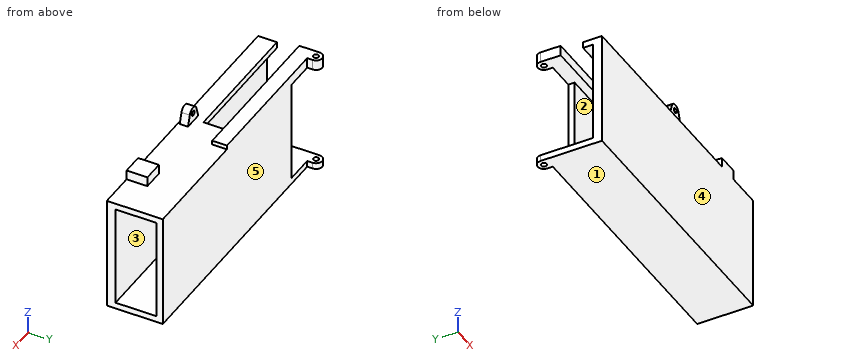
from build123d import *

# Parameters (mm, degrees)
SKETCH_1_W               = 27.5
SKETCH_1_H               = 10.9
SKETCH_1_W_2             = 24.5
SKETCH_1_H_2             = 7.9
EXTRUDE_1_DEPTH          = 66
SKETCH_3_W               = 141.586461115
SKETCH_3_H               = 11.077241851
CUT_EXTRUDE_1_DEPTH      = 50
SKETCH_4_R               = 0.65
EXTRUDE_2_DEPTH          = 27.5
CUT_EXTRUDE_2_DEPTH      = 10
CUT_EXTRUDE_2_DEPTH_BACK = 10
SKETCH_5_W               = 27.947827097
SKETCH_5_H               = 24.5
EXTRUDE_3_DEPTH          = 66
EXTRUDE_START            = -11
SKETCH_9_R               = 0.6
EXTRUDE_5_DEPTH          = 2
SKETCH_10_W              = 33.442715753
SKETCH_10_H              = 5.368535072
CUT_EXTRUDE_3_DEPTH      = 2.6
SKETCH_11_W              = 5
SKETCH_11_H              = 2.3
EXTRUDE_6_DEPTH          = 5
EXTRUDE_START_2          = 1
SKETCH_12_R              = 0.65
EXTRUDE_7_DEPTH          = 1
SKETCH_13_W              = 24.5
SKETCH_13_H              = 0.6
EXTRUDE_8_DEPTH          = 66


with BuildPart() as part:
    # 草图1 → 凸台-拉伸1 (new body)
    with BuildSketch(Plane(origin=(0, 0, 0), x_dir=(0, 0, -1), z_dir=(1, 0, 0))):
        Rectangle(SKETCH_1_W, SKETCH_1_H)
        Rectangle(SKETCH_1_W_2, SKETCH_1_H_2, mode=Mode.SUBTRACT)
    extrude(amount=EXTRUDE_1_DEPTH)

    # 草图3 → 切除-拉伸1 (cut)
    with BuildSketch(Plane.XY.offset(13.75)):
        with Locations((67.57974516, -5.538620926)):
            Rectangle(SKETCH_3_W, SKETCH_3_H)
    extrude(amount=-CUT_EXTRUDE_1_DEPTH, mode=Mode.SUBTRACT)

    # 草图4 → 凸台-拉伸2 (add)
    with BuildSketch(Plane.XY.offset(13.75)):
        with BuildLine():
            Line((0, 6.758945139), (0, 5.45))
            Line((0, 5.45), (3, 5.45))
            Line((3, 5.45), (3, 6.758945139))
            ThreePointArc((3, 6.758945139), (1.5, 8.258945139), (0, 6.758945139))
        make_face()
        with Locations((1.5, 6.758945139)):
            Circle(SKETCH_4_R, mode=Mode.SUBTRACT)
    extrude(amount=-EXTRUDE_2_DEPTH)

    # 草图5 → 切除-拉伸2 (cut, two sides: drawn at the far end of the back side and taken through both)
    with BuildSketch(Plane(origin=(0, 5.45, 0), x_dir=(1, 0, 0), z_dir=(0, 1, 0)).offset(-CUT_EXTRUDE_2_DEPTH_BACK)):
        with Locations((-4.171370472, 0)):
            Rectangle(SKETCH_5_W, SKETCH_5_H)
    extrude(amount=CUT_EXTRUDE_2_DEPTH + CUT_EXTRUDE_2_DEPTH_BACK, mode=Mode.SUBTRACT)

    # 草图6 → 凸台-拉伸3 (add)
    with BuildSketch(Plane(origin=(66, 0, 0), x_dir=(0, 0, -1), z_dir=(1, 0, 0))):
        Polygon((-12.25, 0), (-12.25, -6.49), (12.25, -6.49), (12.25, 0), (13.75, 0), (13.75, -7.99), (-13.75, -7.99), (-13.75, 0), align=None)
    extrude(amount=-EXTRUDE_3_DEPTH)

    # 草图9 → 凸台-拉伸5 (add)
    with BuildSketch(Plane(origin=(0, 5.45, 0), x_dir=(1, 0, 0), z_dir=(0, 1, 0)).offset(EXTRUDE_START)):
        with BuildLine():
            Line((30.537348743, -13.75), (31.33833812, -16.285728508))
            ThreePointArc((31.33833812, -16.285728508), (32.768674372, -17.333911943), (34.199010623, -16.285728508))
            Line((34.199010623, -16.285728508), (35, -13.75))
            Line((35, -13.75), (30.537348743, -13.75))
        make_face()
        with Locations(Location((32.768674372, -15.833911943, 0), (0, 0, 270))):
            Circle(SKETCH_9_R, mode=Mode.SUBTRACT)
    extrude(amount=-EXTRUDE_5_DEPTH)

    # 草图10 → 切除-拉伸3 (cut)
    with BuildSketch(Plane.XY.offset(13.75)):
        with Locations((15.337072277, -0.775945513)):
            Rectangle(SKETCH_10_W, SKETCH_10_H)
    extrude(amount=-CUT_EXTRUDE_3_DEPTH, mode=Mode.SUBTRACT)

    # 草图11 → 凸台-拉伸6 (add)
    with BuildSketch(Plane.XZ.offset(7.99)):
        with Locations((54.86605626, 14.9)):
            Rectangle(SKETCH_11_W, SKETCH_11_H)
    extrude(amount=-EXTRUDE_6_DEPTH)

    # 草图12 → 凸台-拉伸7 (add)
    with BuildSketch(Plane.XY.offset(13.75).offset(EXTRUDE_START_2)):
        with BuildLine():
            Line((32.058430154, 1.908322023), (38.019129527, 1.908322023))
            Line((38.019129527, 1.908322023), (38.019129527, 5.45))
            Line((38.019129527, 5.45), (3, 5.45))
            Line((3, 5.45), (3, 6.758945139))
            ThreePointArc((3, 6.758945139), (1.5, 8.258945139), (0, 6.758945139))
            Line((0, 6.758945139), (0, 1.908322023))
            Line((0, 1.908322023), (32.058430154, 1.908322023))
        make_face()
        with Locations((1.5, 6.758945139)):
            Circle(SKETCH_12_R, mode=Mode.SUBTRACT)
    extrude(amount=-EXTRUDE_7_DEPTH)

    # 草图13 → 凸台-拉伸8 (add)
    with BuildSketch(Plane(origin=(66, 0, 0), x_dir=(0, 0, -1), z_dir=(1, 0, 0))):
        with Locations((0, -6.19)):
            Rectangle(SKETCH_13_W, SKETCH_13_H)
    extrude(amount=-EXTRUDE_8_DEPTH)


solid = part.part
Geometry check sheet. Reference: the model listing, model coordinates, mm. Face numbers are marked on the shaded views. A direction names the side the tool comes from. Give positions to 0.01 mm unless a question says otherwise; leave off trailing zeros. Loops run counter-clockwise (first coordinate to the right, second up) from the corner with the lowest first, then second, coordinate; pieces in that order, holes last. Notation, with made-up numbers: M -15,-10 L -9,-10 A31 ccw -9,20 Z; hole C 19,-37 d8. An arc over 180 degrees is marked long. Write each question's results on one line, items separated by ' | '.
1) Section check B-B, the plane z = 11. Record the boundary of the cut face in (x, y).
Answers follow:
outline: M 0,-7.99 L 66,-7.99 L 66,-5.89 L 0,-5.89 Z; M 9.8,3.95 L 66,3.95 L 66,5.45 L 9.8,5.45 Z
2) Section check A-A, the plane y = 1.25. Record the boundary of the cut face in (x, z).
Answers follow:
outline: M 0,-13.75 L 66,-13.75 L 66,-12.25 L 0,-12.25 Z; M 32.06,12.25 L 66,12.25 L 66,13.75 L 32.06,13.75 Z
3) Gauge pin test, flat ends, axial feed: pin 1 (1.9 mm diameter, centred on x = 13.5, y = 5.5, fed in from +Z); pin 2 (8 mm diameter, centred on x = 11.5, y = -2.5, fed in from +Z); pin 3 (0.7 mm diameter, centred on x = 55, z = 14.5, fed in from +Y); pin 4 (0.8 mm diameter, centred on x = 1.5, y = 6.76, fed in from -Z). Record the tip position at first contact, or that the pin passes through.
Answers follow:
pin 1: z = 14.75 | pin 2: z = 13.75 | pin 3: y = -2.99 | pin 4: through
4) Thickness scan on line 1 (Z direction, x = 53.5, y = 3); line 2 (Y direction, x = 13, z = -11); line 3 (Z direction, x = 12.5, y = 2.75). Record the ranges inside material, lowest first.
Answers follow:
line 1: -13.75 to -12.25, 12.25 to 13.75 | line 2: -7.99 to -5.89, 3.95 to 5.45 | line 3: -13.75 to -12.25, 12.25 to 14.75
5) Section check C-C, the plane x = 51. Record the boundary of the cut face in (y, z).
Answers follow:
outline: M -7.99,-13.75 L 5.45,-13.75 L 5.45,13.75 L -7.99,13.75 Z; hole M -5.89,-12.25 L 3.95,-12.25 L 3.95,12.25 L -5.89,12.25 Z
6) Release check for a two-part mould opening along Y. For the marked faces 3, 4 and 5 record: +Y half, -Y half, draft (parallel to the pull), parting line (faces both ways), or undercut.
Answers follow:
face 3: undercut | face 4: -Y half | face 5: +Y half
7) Section check D-D, the plane x = 1.5. Record the boundary of the cut face in (y, z).
Answers follow:
outline: M -7.99,-13.75 L 6.11,-13.75 L 6.11,-12.25 L -5.89,-12.25 L -5.89,12.25 L -3.46,12.25 L -3.46,13.75 L -7.99,13.75 Z; M 1.91,12.25 L 6.11,12.25 L 6.11,14.75 L 1.91,14.75 Z; M 7.41,-13.75 L 8.26,-13.75 L 8.26,-12.25 L 7.41,-12.25 Z; M 7.41,12.25 L 8.26,12.25 L 8.26,14.75 L 7.41,14.75 Z
8) Tool access check on the marked faces 1 and 2. Record the directions out of +Z, -Z, +X, -X, +Y, -Y that give a thin tool (end or side, any length) a straight path to the whole face; none if there is none.
Answers follow:
face 1: -Z, +X, -X, +Y, -Y | face 2: +X, -X
